Geometry check sheet. Reference: the model listing, model coordinates, mm. Give positions to 0.01 mm unless a question says otherwise; leave off trailing zeros. Write each loop counter-clockwise with the first axis right and the second up, starting at its lowest first coordinate (ties: lowest second). Pieces come first, ordered by that corner, then holes. Notation, with made-up numbers: M 52,22.25 L 76,22.25 A26 cw 76,39.25 Z; hole C -19,15 d10. An arc over 180 degrees is marked long. One line per item, written item: value. Start each with the question number.
1. Cross-section at A-A on x = 0. Count the separate pieces of the cut face and the enclosed holes in it, then the cut area to 3 significant figures.
2. Cross-section at C-C on y = -24. Record the cut outline in (x, z) (3 decimals).
3. Gauge pin test, flat ends, axial feed: pin 1 (6 mm diameter, centred on x = 25.02, y = 25.01, fed in from +Z); pin 2 (8 mm diameter, centred on x = 0, y = 0, fed in from +Z); pin 3 (1 mm diameter, centred on x = 3, y = 10.5, fed in from +Z). Record the tip position at first contact, or that the pin passes through.
4. Scan lines: line 1 (Y direction, x = 26, z = 1.25) (3 decimals); line 2 (Y direction, x = 12.5, z = 6.25) (3 decimals); line 3 (Y direction, x = 11, z = 5.25) (3 decimals). Record each from-to range of solid material in increasing order.
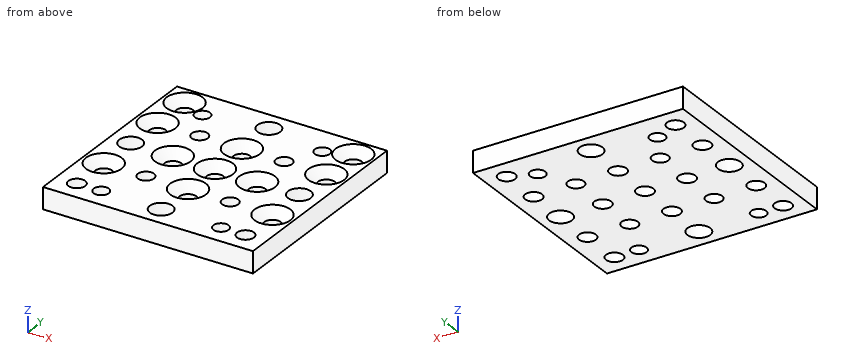
from build123d import *

# Parameters (mm, degrees)
SKETCH1_W           = 62.23
SKETCH1_H           = 62.23
SKETCH1_R           = 2.5
SKETCH1_R_2         = 2.25
BOSS_EXTRUDE1_DEPTH = 6.35
CHAMFER1_SIZE       = 2.8
SKETCH2_R           = 3.3655
SKETCH2_R_2         = 2.3876
CUT_EXTRUDE2_DEPTH  = 45.459070503


with BuildPart() as part:
    # Sketch1 → Boss-Extrude1 (new body)
    with BuildSketch(Plane.XY):
        Rectangle(SKETCH1_W, SKETCH1_H)
        with Locations((25.019, 25.0063)):
            Circle(SKETCH1_R, mode=Mode.SUBTRACT)
        with Locations((25.019, 12.4968)):
            Circle(SKETCH1_R, mode=Mode.SUBTRACT)
        with Locations((25.019, -12.4968)):
            Circle(SKETCH1_R, mode=Mode.SUBTRACT)
        with Locations((25.019, -24.9936)):
            Circle(SKETCH1_R, mode=Mode.SUBTRACT)
        with Locations((12.4968, 0)):
            Circle(SKETCH1_R, mode=Mode.SUBTRACT)
        with Locations((0, 12.4968)):
            Circle(SKETCH1_R, mode=Mode.SUBTRACT)
        Circle(SKETCH1_R, mode=Mode.SUBTRACT)
        with Locations((0, -12.4968)):
            Circle(SKETCH1_R, mode=Mode.SUBTRACT)
        with Locations((-24.9936, -24.9936)):
            Circle(SKETCH1_R, mode=Mode.SUBTRACT)
        with Locations((-24.9936, -12.4968)):
            Circle(SKETCH1_R, mode=Mode.SUBTRACT)
        with Locations((-12.4968, 0)):
            Circle(SKETCH1_R, mode=Mode.SUBTRACT)
        with Locations((-24.9936, 25.0063)):
            Circle(SKETCH1_R, mode=Mode.SUBTRACT)
        with Locations((-24.9936, 12.4968)):
            Circle(SKETCH1_R, mode=Mode.SUBTRACT)
        with Locations((-17.75, 22)):
            Circle(SKETCH1_R_2, mode=Mode.SUBTRACT)
        with Locations((17.75, 22)):
            Circle(SKETCH1_R_2, mode=Mode.SUBTRACT)
        with Locations((17.75, -25)):
            Circle(SKETCH1_R_2, mode=Mode.SUBTRACT)
        with Locations((-17.75, -25)):
            Circle(SKETCH1_R_2, mode=Mode.SUBTRACT)
    extrude(amount=BOSS_EXTRUDE1_DEPTH)

    # Chamfer1
    chamfer1_edges = [part.edges().sort_by_distance(p)[0] for p in [
        (22.519, 25.0063, 6.35),
        (22.519, 12.4968, 6.35),
        (22.519, -12.4968, 6.35),
        (9.9968, 0, 6.35),
        (-2.5, 12.4968, 6.35),
        (-2.5, 0, 6.35),
        (-2.5, -12.4968, 6.35),
        (-27.4936, -12.4968, 6.35),
        (-14.9968, 0, 6.35),
        (-27.4936, 25.0063, 6.35),
        (-27.4936, 12.4968, 6.35),
    ]]
    chamfer(chamfer1_edges, length=CHAMFER1_SIZE)

    # Sketch2 → Cut-Extrude2 (cut, through all)
    with BuildSketch(Plane.XY.offset(6.35)):
        with Locations((0, -24.9936)):
            Circle(SKETCH2_R)
        with Locations((0, 25.019)):
            Circle(SKETCH2_R)
        with Locations((12.4968, 12.4968)):
            Circle(SKETCH2_R_2)
        with Locations((-12.4968, 12.4968)):
            Circle(SKETCH2_R_2)
        with Locations((-12.4968, -12.4968)):
            Circle(SKETCH2_R_2)
        with Locations((12.4968, -12.4968)):
            Circle(SKETCH2_R_2)
        with Locations((25.019, 0)):
            Circle(SKETCH2_R)
        with Locations((-24.9936, 0)):
            Circle(SKETCH2_R)
    extrude(amount=-CUT_EXTRUDE2_DEPTH, mode=Mode.SUBTRACT)


solid = part.part
Report:
1. separate pieces: 6
1. enclosed holes: 0
1. area: 191 mm^2
2. outline: M -31.115,0 L -27.288,0 L -27.288,6.35 L -31.115,6.35 Z; M -22.7,0 L -19.766,0 L -19.766,6.35 L -22.7,6.35 Z; M -15.734,0 L -3.215,0 L -3.215,6.35 L -15.734,6.35 Z; M 3.215,0 L 15.734,0 L 15.734,6.35 L 3.215,6.35 Z; M 19.766,0 L 22.725,0 L 22.725,6.35 L 19.766,6.35 Z; M 27.313,0 L 31.115,0 L 31.115,6.35 L 27.313,6.35 Z
3. pin 1: stops at z = 4.05
3. pin 2: stops at z = 5.05
3. pin 3: stops at z = 5.15
4. line 1: y = -31.115 to -27.293, -22.694 to -14.796, -10.197 to -3.219, 3.219 to 10.197, 14.796 to 22.707, 27.306 to 31.115
4. line 2: y = -31.115 to -14.884, -10.109 to -5.2, 5.2 to 10.109, 14.884 to 31.115
4. line 3: y = -31.115 to -14.357, -10.637 to -3.924, 3.924 to 10.637, 14.357 to 31.115
